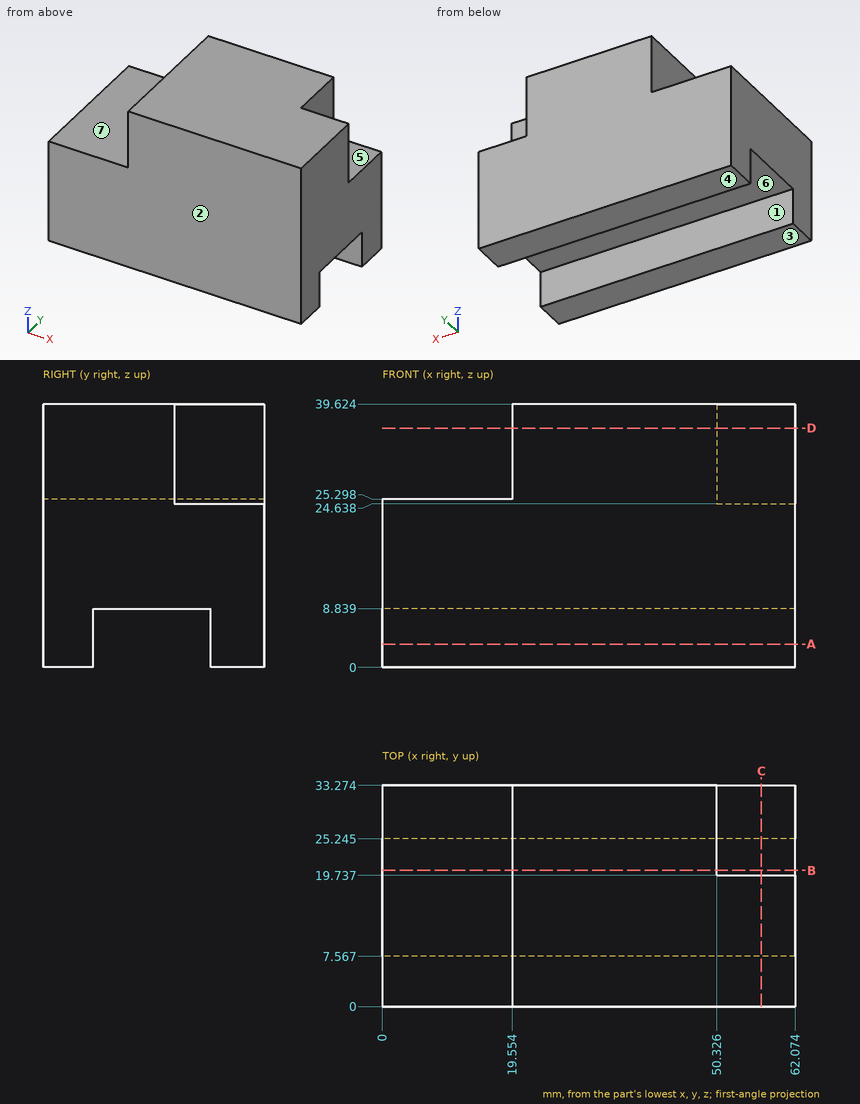
Source: three-view drawing plus pictorial views. Frame: mm from the lowest corner of the part. A direction names the side the tool comes from. Coordinates: 2 decimals unless noted, no trailing zeros. Order: outer loops, then holes, each group sorted by start corner. A loop starts at its lowest first (then second) coordinate and runs counter-clockwise, first axis right, second up. Notation, with made-up numbers: (13.5, -31) -> (58.5, -31) arc R22 cw to (58.5, 1) -> close; hole circle Ø3 at (-33, 62.5). An arc over 180 degrees is marked (long way). Write item = value, one per line.
(1) Pull-direction query (Y, two-part tool) for the marked faces 1, 2 and 3; classes: pulls with the +Y half, pulls with the -Y half, needs draft (parallel to the pull), parting line crosses it, or undercut.
Solved:
face_1 = undercut
face_2 = pulls with the -Y half
face_3 = needs draft
(2) Cut plane A-A on z = 3.5. Return loops of the section in (x, y) (1 decimal).
Solved:
outline = (0, 0) -> (62.1, 0) -> (62.1, 7.6) -> (0, 7.6) -> close; (0, 25.2) -> (62.1, 25.2) -> (62.1, 33.3) -> (0, 33.3) -> close
(3) Cut plane D-D on z = 36. Return loops of the section in (x, y).
Solved:
outline = (19.55, 0) -> (62.07, 0) -> (62.07, 19.74) -> (50.33, 19.74) -> (50.33, 33.27) -> (19.55, 33.27) -> close
(4) Line query: line 1 (Y direction, x = 5.5, z = 8) (1 decimal); line 2 (X direction, y = 18, z = 34); line 3 (Y direction, x = 50.5, z = 36.5). Output: solid intervals per line, ascending.
Solved:
line_1 = 0 to 7.6, 25.2 to 33.3
line_2 = 19.55 to 62.07
line_3 = 0 to 19.74
(5) Cut plane B-B on y = 20.5. Return loops of the section in (x, z), plus the area to 3 significant figures.
Solved:
outline = (0, 8.84) -> (62.07, 8.84) -> (62.07, 24.64) -> (50.33, 24.64) -> (50.33, 39.62) -> (19.55, 39.62) -> (19.55, 25.3) -> (0, 25.3) -> close
area = 1,450 mm²
(6) Access query for the marked faces 4, 5, 6 and 7. Directions: +Z, -Z, +X, -X, +Y, -Y. A direction counts if a zero-diameter tool reaches every point of the face in a straight line with its end or side. Return the directions, or none.
Solved:
face_4 = -Z, +X, -X, +Y, -Y
face_5 = +Z, +X, +Y
face_6 = -Z, +X, -X
face_7 = +Z, -X, +Y, -Y
(7) Pin query (flat end, axial travel): pin 1 Ø4 at (y, z) = (29.5, 30.5) entering from +X; pin 2 Ø6 at (x, y) = (30, 22.5) entering from -Z; pin 3 Ø3.5 at (x, y) = (59, 25.5) entering from +Z; pin 4 Ø3.5 at (x, z) = (58, 31) entering from +Y. Return the tip coordinate at first contact, or that it passes through.
Solved:
pin_1 = 50.33
pin_2 = 0
pin_3 = 24.64
pin_4 = 19.74
(8) Cut plane C-C on x = 57. Return loops of the section in (y, z) (1 decimal), plus the area to 3 significant figures.
Solved:
outline = (0, 0) -> (7.6, 0) -> (7.6, 8.8) -> (25.2, 8.8) -> (25.2, 0) -> (33.3, 0) -> (33.3, 24.6) -> (19.7, 24.6) -> (19.7, 39.6) -> (0, 39.6) -> close
area = 959 mm²
